Input: part model. Units: mm. Frame: model coordinates. A direction names the side the tool comes from. Coordinates: 2 decimals unless noted, no trailing zeros. Loops run counter-clockwise (first coordinate to the right, second up) from the corner with the lowest first, then second, coordinate; pieces in that order, holes last. Notation, with made-up numbers: (66, -4.75) - (86, -4.75) arc R23 cw to (86, 30.25) - close; hole circle Ø9 at (-12.75, 76). An arc over 180 degrees is marked (long way). Use a Markdown table: item, result. Add a question column.
1. Contact query for flat-ended pins moving along their axis: P1, Ø1.5, axis at y = 17.5, z = -12, coming from the +X side; P2, Ø12, axis at x = 9, y = 8.5, coming from the -Z side; P3, Ø4, axis at y = -0.5, z = 1, coming from the -X side. Output: stop coordinate, or through.
2. Ray query, L1, parallel to Z at x = -0.8, y = 12; L2, parallel to X at y = 14, z = 19; L3, parallel to Z at x = 11, y = 27. Return the intervals inside material, ascending. Write a range as [from, to].
3. Section query D-D on y = -7.5. Return the cut outline in (x, z).
4. Section query B-B on x = 0. State how many separate pieces and enclosed holes the cut face has, then the cut area to 3 significant figures.
5. Section query C-C on y = 25.5. Return the cut outline in (x, z).
6. Section query A-A on y = 12. Return the cut outline in (x, z).
7. Access query for faces 1 (the face through (1.5, 16, -18)), 2 (the face through (-1.5, 16, -18)), 3 (the face through (-1.5, 16, 18)), 4 (the face through (0, 8, -14)). Directions: +Z, -Z, +X, -X, +Y, -Y. A direction counts if a zero-diameter tool reaches every point of the face in a straight line with its end or side. Return the directions, or none.
8. Draft query along X for faces 5 (the face through (1.5, 16, 18)), 6 (the face through (3.74, 12.34, 9.01)), 7 (the face through (-0.744, -15.219, 2.364)), 8 (the face through (2.68, 3.22, 6.47)). Return one class per face: released by +X, released by -X, zero draft, split by the parting line, or undercut.
```python
from build123d import *

# Parameters (mm, degrees)
F2_R     = 2
F3_DEPTH = 1.5
F4_R     = 1
F5_R     = 5
F6_R     = 5
F7_R     = 3


with BuildPart() as f1:
    # F0 (on Right) → F1 (revolve)
    with BuildSketch(Plane.YZ):
        Polygon((-30, 2.004988), (-30, 1), (0, 4), (15, 10.994615), (30, 17.98923), (30, 21.299364), (15, 14.304749), (0, 5.004988), align=None)
    revolve(axis=Axis((0, -9.670749, 0), (0, -1, 0)))

    # F2 (on Right) → F3 (join, symmetric)
    with BuildSketch(Plane.YZ):
        Polygon((8, 9.105201), (30, 21.3), (8, 21.3), align=None)
        with Locations((12, 17.3)):
            Circle(F2_R, mode=Mode.SUBTRACT)
        Polygon((8, -21.3), (30, -21.3), (8, -9.105201), align=None)
        with Locations((12, -17.3)):
            Circle(F2_R, mode=Mode.SUBTRACT)
    extrude(amount=F3_DEPTH, both=True)

    # F4
    f4_edges = [f1.edges().sort_by_distance(p)[0] for p in [
        (0, -30, -2.004988),
    ]]
    fillet(f4_edges, radius=F4_R)

    # F5
    f5_edges = [f1.edges().sort_by_distance(p)[0] for p in [
        (0, 0, -5.004988),
    ]]
    fillet(f5_edges, radius=F5_R)

    # F6
    f6_edges = [f1.edges().sort_by_distance(p)[0] for p in [
        (0, 0, -4),
    ]]
    fillet(f6_edges, radius=F6_R)

    # F7
    f7_edges = [f1.edges().sort_by_distance(p)[0] for p in [
        (0, 8, 21.3),
        (0, 8, -21.3),
    ]]
    fillet(f7_edges, radius=F7_R)


solid = f1.part
```
Resolved:
| question | item | result |
|---|---|---|
| 1 | P1 | x = 10.77 |
| 1 | P2 | z = -12.11 |
| 1 | P3 | x = -5.88 |
| 2 | L1 | [-21.3, -19.3], [-15.3, -9.56], [9.56, 15.3], [19.3, 21.3] |
| 2 | L2 | [-1.5, 1.5] |
| 2 | L3 | [-16.58, -12.42], [12.42, 16.58] |
| 3 | outline | circle Ø8.51 at (0, 0); hole circle Ø6.5 at (0, 0) |
| 4 | separate pieces | 2 |
| 4 | enclosed holes | 2 |
| 4 | area | 428 mm² |
| 5 | outline | (-1.5, -21.3) - (1.5, -21.3) - (1.5, -19.14) arc R19.2 ccw to (1.5, 19.14) - (1.5, 21.3) - (-1.5, 21.3) - (-1.5, 19.14) arc R19.2 ccw to (-1.5, -19.14) - close; hole circle Ø31.78 at (0, 0) |
| 6 | outline | (-1.5, -21.3) - (1.5, -21.3) - (1.5, -19.3) - (-1.5, -19.3) - close; (-1.5, -15.3) - (1.5, -15.3) - (1.5, -12.35) arc R12.44 ccw to (1.5, 12.35) - (1.5, 15.3) - (-1.5, 15.3) - (-1.5, 12.35) arc R12.44 ccw to (-1.5, -12.35) - close; (-1.5, 19.3) - (1.5, 19.3) - (1.5, 21.3) - (-1.5, 21.3) - close; hole circle Ø19.19 at (0, 0) |
| 7 | face 1 | -Z, +X, -Y |
| 7 | face 2 | -Z, -X, -Y |
| 7 | face 3 | +Z, -X, -Y |
| 7 | face 4 | -Z, +X, -X, -Y |
| 8 | face 5 | released by +X |
| 8 | face 6 | undercut |
| 8 | face 7 | undercut |
| 8 | face 8 | split by the parting line |
